Design review of the part built by this model. Coordinates are the model's own, in mm. Face numbers are marked on the shaded views. A direction names the side the tool comes from. Round coordinates to 2 decimals unless told otherwise and drop trailing zeros. Order: outer loops, then holes, each group sorted by start corner. A loop starts at its lowest first (then second) coordinate and runs counter-clockwise, first axis right, second up. Notation, with made-up numbers: (-22, -34.75) - (4, -34.75) arc R27 ccw to (4, -1.75) - close; hole circle Ø6 at (69, -13). An arc over 180 degrees is marked (long way). Write item = value, one per line.
from build123d import *

# Parameters (mm, degrees)
SKETCH1_W           = 10
SKETCH1_H           = 8
BOSS_EXTRUDE1_DEPTH = 11
SKETCH2_W           = 2
SKETCH2_H           = 1
SKETCH2_W_2         = 3
SKETCH2_H_2         = 2
CUT_EXTRUDE1_DEPTH  = 11
SKETCH3_W           = 4
SKETCH3_H           = 2
CUT_EXTRUDE2_DEPTH  = 2
CUT_EXTRUDE3_DEPTH  = 4
SKETCH5_W           = 2
SKETCH5_H           = 1
CUT_EXTRUDE4_DEPTH  = 5
SKETCH6_W           = 2
SKETCH6_H           = 5
CUT_EXTRUDE5_DEPTH  = 9
CUT_EXTRUDE6_DEPTH  = 7
CUT_EXTRUDE7_DEPTH  = 7
CUT_EXTRUDE8_DEPTH  = 2


with BuildPart() as part:
    # Sketch1 → Boss-Extrude1 (new body)
    with BuildSketch(Plane.XY):
        with Locations((5, 4)):
            Rectangle(SKETCH1_W, SKETCH1_H)
    extrude(amount=BOSS_EXTRUDE1_DEPTH)

    # Sketch2 → Cut-Extrude1 (cut)
    with BuildSketch(Plane.ZY):
        with Locations((1, 7.5)):
            Rectangle(SKETCH2_W, SKETCH2_H)
        with Locations((9.5, 7)):
            Rectangle(SKETCH2_W_2, SKETCH2_H_2)
    extrude(amount=-CUT_EXTRUDE1_DEPTH, mode=Mode.SUBTRACT)

    # Sketch3 → Cut-Extrude2 (cut)
    with BuildSketch(Plane.XY.offset(11)):
        with Locations((5, 5)):
            Rectangle(SKETCH3_W, SKETCH3_H)
    extrude(amount=-CUT_EXTRUDE2_DEPTH, mode=Mode.SUBTRACT)

    # Sketch4 → Cut-Extrude3 (cut)
    with BuildSketch(Plane.XY.offset(11)):
        Polygon((3, 4), (2, 3), (2, 8), (7, 8), align=None)
    extrude(amount=-CUT_EXTRUDE3_DEPTH, mode=Mode.SUBTRACT)

    # Sketch5 → Cut-Extrude4 (cut)
    with BuildSketch(Plane.XY.offset(7)):
        Polygon((6, 7), (7, 8), (2, 8), (2, 7), align=None)
        with Locations((1, 7.5)):
            Rectangle(SKETCH5_W, SKETCH5_H)
    extrude(amount=-CUT_EXTRUDE4_DEPTH, mode=Mode.SUBTRACT)

    # Sketch6 → Cut-Extrude5 (cut)
    with BuildSketch(Plane.XY.offset(11)):
        with Locations((1, 5.5)):
            Rectangle(SKETCH6_W, SKETCH6_H)
    extrude(amount=-CUT_EXTRUDE5_DEPTH, mode=Mode.SUBTRACT)

    # Sketch7 → Cut-Extrude6 (cut)
    with BuildSketch(Plane.XY.offset(7)):
        Polygon((3, 7), (0, 4), (0, 7), align=None)
    extrude(amount=-CUT_EXTRUDE6_DEPTH, mode=Mode.SUBTRACT)

    # Sketch9 → Cut-Extrude7 (cut)
    with BuildSketch(Plane(origin=(0, 3, 0), x_dir=(1, 0, 0), z_dir=(0, 1, 0))):
        Polygon((0, -2), (1, -3), (1, -11), (0, -11), align=None)
    extrude(amount=-CUT_EXTRUDE7_DEPTH, mode=Mode.SUBTRACT)

    # Sketch10 → Cut-Extrude8 (cut)
    with BuildSketch(Plane.XZ):
        Polygon((1, 3), (2, 4), (7.595103791, 4), (7.595103791, 9.328283849), (7.595103791, 11), (4, 11), (4, 10), (1, 10), (1, 4.286480229), align=None)
    extrude(amount=-CUT_EXTRUDE8_DEPTH, mode=Mode.SUBTRACT)


solid = part.part
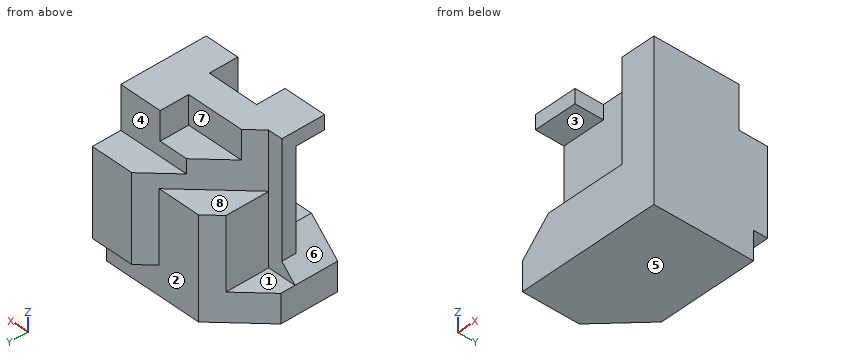
1) We need section B-B on z = 3.5. Write out the cut boundary in (x, y), and give its area (3 significant figures).
Findings:
outline = (1, 2) - (1.5, 2) - (1.5, 0) - (10, 0) - (10, 8) - (7, 8) - (6, 7) - (3, 7) - (2, 6) - (2, 3) - (1, 3) - close
area = 61.0 mm^2
2) We need section D-D on y = 3.75. Write out the cut boundary in (x, z).
Findings:
outline = (0, 0) - (10, 0) - (10, 11) - (2.75, 11) - (2.75, 7) - (2, 7) - (2, 2) - (0, 2) - close
3) Clearance check with flat-ended pins moving along their axes: pin 1 Ø2 at (x, y) = (6, 1.5) entering from +Z; pin 2 Ø4 at (x, z) = (1.5, 2.5) entering from +Y; pin 3 Ø2.5 at (y, z) = (4.5, 3.5) entering from -X; pin 4 Ø0.6 at (y, z) = (5, 10) entering from -X. State where each tip first meets the part, or that it passes through.
Findings:
pin_1 = 11
pin_2 = 7
pin_3 = 2
pin_4 = 7
4) We need section A-A on y = 1.5. Write out the cut boundary in (x, z).
Findings:
outline = (0, 0) - (10, 0) - (10, 11) - (7.6, 11) - (7.6, 4) - (2, 4) - (0, 2) - close; (1, 10) - (4, 10) - (4, 11) - (1, 11) - close
5) The part is to be moulded in two halves that separate along Z. For the marked faces 6, 7 and 8, say which applies: released by +Z, released by -Z, zero draft, split by the parting line, or undercut.
Findings:
face_6 = undercut
face_7 = zero draft
face_8 = released by +Z
6) For the marked faces 1, 2, 3, 4 and 5, list the 3-axis set-ups (+Z, -Z, +X, -X, +Y, -Y) from which the entire face can be reached by the end or side of a thin tool; tool diameter is ignored.
Findings:
face_1 = +Z, -X, +Y
face_2 = -Z, -X, +Y
face_3 = -X, -Y
face_4 = +Z, +X, -X, +Y
face_5 = -Z, +X, -X, +Y, -Y
7) To check wall thickness, follow L1, parallel to X at y = 0.75, z = 3; L2, parallel to Y at x = 9, z = 10.75; L3, parallel to X at y = 4.75, z = 6. State the ranges of each line that lie inside material, in increasing order. Write a range as from..to.
Findings:
L1 = 1..10
L2 = 0..6
L3 = 2..10
8) We need section C-C on x = 6.5. Write out the cut boundary in (y, z), and give its area (3 significant figures).
Findings:
outline = (0, 0) - (7, 0) - (7, 2) - (7.5, 2) - (7.5, 8) - (6, 8) - (6, 9) - (4, 9) - (4, 11) - (2, 11) - (2, 4) - (0, 4) - close
area = 59.0 mm^2
